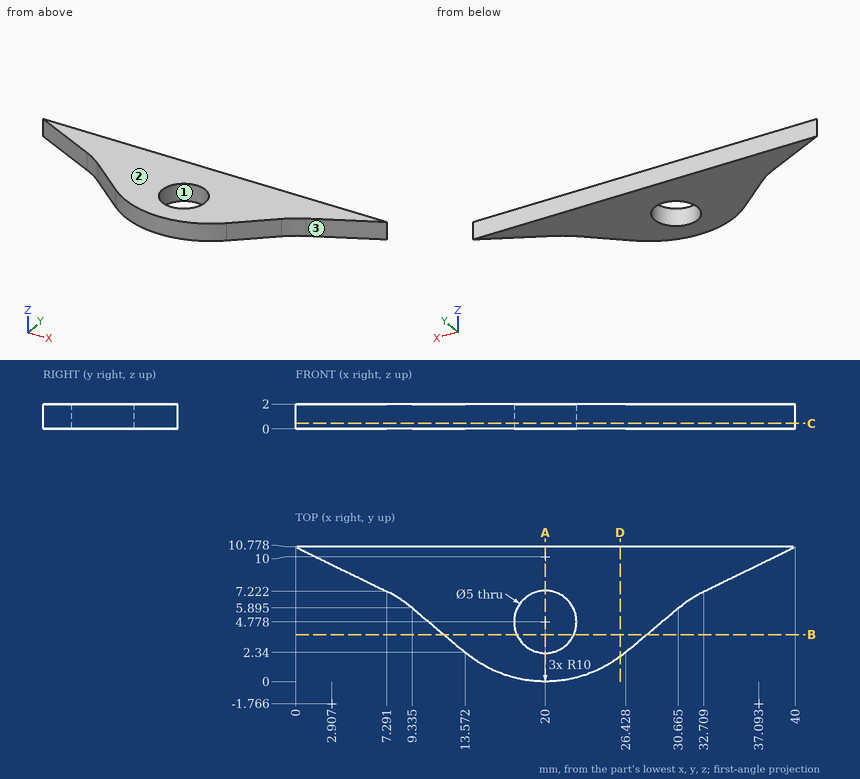
The drawing under review shows one solid part. Ordinate dimensions are in mm from its lowest x, y, z. Give positions to 0.01 mm unless a question says otherwise; leave off trailing zeros. Write each loop counter-clockwise with the first axis right and the second up, starting at its lowest first coordinate (ties: lowest second). Pieces come first, ordered by that corner, then holes. Notation, with made-up numbers: (37.5, 49.25) - (60.5, 49.25) arc R38 ccw to (60.5, 87.25) - close; hole circle Ø10 at (66, 53.5). An arc over 180 degrees is marked (long way). Answer in a Markdown table with one row per item. Add a question column.
1. Draft analysis for pull direction Y (two halves, no side actions). For the marked faces 1, 2 and 3, state which applies: +Y half, -Y half, draft (parallel to the pull), parting line (faces both ways), or undercut.
2. We need section A-A on x = 20. Write out the cut boundary in (y, z).
3. Wall thickness on line 1 along Y through (x, z) = (20, 1.15); line 2 along Y through (x, z) = (26, 0.15); line 3 along Y through (x, z) = (18.5, 1.6) (1 decimal): over which ranges is each line inside the solid? List them lowest first. Write a range as [from, to].
4. We need section D-D on x = 26. Write out the cut boundary in (y, z).
5. We need section B-B on y = 3.75. Write out the cut boundary in (x, z).
6. Insertion check: P1, Ø3, axis at x = 25, y = 4.5, coming from the -Z side. The pin has a flat end and moves straight along its axis. Give the tip position at first contact, or say it passes through.
7. We need section C-C on z = 0.45. Write out the cut boundary in (x, y) (1 decimal), then the cut area to 3 significant figures.
Ans:
| question | item | result |
|---|---|---|
| 1 | face 1 | undercut |
| 1 | face 2 | draft |
| 1 | face 3 | -Y half |
| 2 | outline | (0, 0) - (2.28, 0) - (2.28, 2) - (0, 2) - close; (7.28, 0) - (10.78, 0) - (10.78, 2) - (7.28, 2) - close |
| 3 | line 1 | y = [0, 2.28], [7.28, 10.78] |
| 3 | line 2 | y = [2, 10.78] |
| 3 | line 3 | y = [0.1, 2.8], [6.8, 10.8] |
| 4 | outline | (2, 0) - (10.78, 0) - (10.78, 2) - (2, 2) - close |
| 5 | outline | (11.89, 0) - (17.72, 0) - (17.72, 2) - (11.89, 2) - close; (22.28, 0) - (28.11, 0) - (28.11, 2) - (22.28, 2) - close |
| 6 | P1 | stops at z = 0 |
| 7 | outline | (0, 10.8) - (7.3, 7.2) arc R10 cw to (9.3, 5.9) - (13.6, 2.3) arc R10 ccw to (26.4, 2.3) - (30.7, 5.9) arc R10 cw to (32.7, 7.2) - (40, 10.8) - close; hole circle Ø5 at (20, 4.8) |
| 7 | area | 209 mm^2 |
